```python
from build123d import *
from OCP.BRepFilletAPI import BRepFilletAPI_MakeChamfer

# Parameters (mm, degrees)
CHANFREIN1_SIZE    = 1
CHANFREIN1_SIZE2   = 0.808473415
CHANFREIN1_SIZE2_2 = 1.458524649


with BuildPart() as part:
    # Esquisse1 → Révolution1 (revolve)
    with BuildSketch(Plane.XY, mode=Mode.PRIVATE) as r_volution1_sk:
        Polygon((0, 21.5), (0, 25.25), (17.5, 25.25), (18, 24.75), (23.47253806, 24.75), (50.5, 17), (50.5, 11.5), (17.369562784, 21), (15.869562784, 22.5), (7, 22.5), (7, 21.5), align=None)
    revolve(r_volution1_sk.sketch.rotate(Axis((0, 0, 0), (-1, 0, 0)), 90), axis=Axis((0, 0, 0), (-1, 0, 0)))

    # Chanfrein1: one chamfer whose edges measure the first distance from different faces: ONE call of the kernel's chamfer builder (chamfer() names one face for all edges)
    chanfrein1_edges_1 = [part.edges().sort_by_distance(p)[0] for p in [
        (0, 0, 21.5),
    ]]
    chanfrein1_edges_2 = [part.edges().sort_by_distance(p)[0] for p in [
        (50.5, 0, 11.5),
    ]]
    chanfrein1_side_2 = [part.faces().sort_by_distance(p)[0] for p in [
        (50.5, 0, 16.519167389),
    ]]
    chanfrein1_edges_3 = [part.edges().sort_by_distance(p)[0] for p in [
        (50.5, 0, 17),
    ]]
    chanfrein1_side_3 = [part.faces().sort_by_distance(p)[0] for p in [
        (36.98626903, 0, 20.875),
    ]]
    chanfrein1 = BRepFilletAPI_MakeChamfer(part.part.solid().wrapped)
    for e in chanfrein1_edges_1:
        chanfrein1.Add(CHANFREIN1_SIZE, e.wrapped)
    for e in chanfrein1_edges_2:
        chanfrein1.Add(CHANFREIN1_SIZE, CHANFREIN1_SIZE2, e.wrapped, chanfrein1_side_2[0].wrapped)  # the first distance lies on this face
    for e in chanfrein1_edges_3:
        chanfrein1.Add(CHANFREIN1_SIZE, CHANFREIN1_SIZE2_2, e.wrapped, chanfrein1_side_3[0].wrapped)  # the first distance lies on this face
    add(Compound.cast(chanfrein1.Shape()), mode=Mode.REPLACE)


solid = part.part
```
Verification items for the finished model (mm, model axes). A direction names the side the tool comes from. Coordinates: 2 decimals unless noted, no trailing zeros. Order: outer loops, then holes, each group sorted by start corner. A loop starts at its lowest first (then second) coordinate and runs counter-clockwise, first axis right, second up. Notation, with made-up numbers: (33, 71) - (52, 71) arc R19 cw to (52, 87) - close; hole circle Ø11 at (-20.75, 76). An arc over 180 degrees is marked (long way). Return JSON: item names as keys, results as strings.
(1) Thickness scan on line 1 along Y through (x, z) = (10.25, 0); line 2 along Y through (x, z) = (46, -5); line 3 along Z through (x, y) = (44.5, -6). Record the ranges inside material, lowest first.
Filled sheet:
{"line 1": "y = -25.25 to -22.5, 22.5 to 25.25", "line 2": "y = -17.59 to -11.77, 11.77 to 17.59", "line 3": "z = -17.73 to -11.78, 11.78 to 17.73"}
(2) Section check D-D, the plane x = 24.5. Record the cut outline in (y, z).
Filled sheet:
{"outline": "circle Ø48.91 at (0, 0); hole circle Ø37.91 at (0, 0)"}
(3) Mould release check, pull along Z, two halves, no side actions. Record for faces 1 (the flat face through (0, 15, -17)), 2 (the cylindrical face through (3.958, -21.317, 2.799)), 3 (the cylindrical face through (8.87, 15.36, 20.04)): pulls with the +Z half, pulls with the -Z half, needs draft (parallel to the pull), parting line crosses it, or undercut.
Filled sheet:
{"face 1": "needs draft", "face 2": "undercut", "face 3": "parting line crosses it"}
(4) Go/stop test with flat-tipped pins: pin 1 (1 mm diameter, centred on x = 30.5, z = 3, fed in from +Y); pin 2 (3 mm diameter, centred on x = 11.5, z = -10, fed in from -Y); pin 3 (6 mm diameter, centred on x = 21.5, y = -7, fed in from +Z); pin 4 (13.5 mm diameter, centred on y = 3, z = 2.5, fed in from +X). Record where each tip stops, or that it passes through.
Filled sheet:
{"pin 1": "stops at y = 22.69", "pin 2": "stops at y = -23.78", "pin 3": "stops at z = 24.42", "pin 4": "passes through"}
(5) Section check A-A, the plane y = 0. Record the cut outline in (x, z), and give its area (3 significant figures).
Filled sheet:
{"outline": "(0, -25.25) - (17.5, -25.25) - (18, -24.75) - (23.47, -24.75) - (49.54, -17.28) - (50.5, -15.54) - (50.5, -12.5) - (49.72, -11.72) - (17.37, -21) - (15.87, -22.5) - (7, -22.5) - (7, -21.5) - (1, -21.5) - (0, -22.5) - close; (0, 22.5) - (1, 21.5) - (7, 21.5) - (7, 22.5) - (15.87, 22.5) - (17.37, 21) - (49.72, 11.72) - (50.5, 12.5) - (50.5, 15.54) - (49.54, 17.28) - (23.47, 24.75) - (18, 24.75) - (17.5, 25.25) - (0, 25.25) - close", "area": "463 mm^2"}
(6) Section check C-C, the plane x = 13.5. Record the cut outline in (y, z), and give its area (3 significant figures).
Filled sheet:
{"outline": "circle Ø50.5 at (0, 0); hole circle Ø45 at (0, 0)", "area": "413 mm^2"}
(7) Access from +Z, -Z, +X, -X, +Y, -Y to the whole of each face (thin tool, end or side, straight path). Record for faces 4 (the flat face through (50.5, -13, -1)), 5 (the flat face through (7, 2, -22)), 6 (the cylindrical face through (20.77, -16.73, 18.24)).
Filled sheet:
{"face 4": "+Z, -Z, +X, +Y, -Y", "face 5": "none", "face 6": "+X"}
